from build123d import *

# Parameters (mm, degrees)
F1_DEPTH             = 20
F2_R                 = 5
F3_R                 = 1.99999
F6_D                 = 5
F6_DEPTH             = 10
F6_CSINK_D           = 10
F6_CSINK_ANGLE       = 90
F6_TIP               = 1.5021515476
F6_ON_F5_D           = 5
F6_ON_F5_DEPTH       = 10
F6_ON_F5_CSINK_D     = 10
F6_ON_F5_CSINK_ANGLE = 90
F6_ON_F5_TIP         = 1.5021515476
F7_D                 = 10
F7_DEPTH             = 49.0010001
F7_ON_F5_D           = 10
F7_ON_F5_DEPTH       = 49.0010001


# Not quite as in the source:
# - a fillet or chamfer is up to 0.001 mm smaller than in the source, because OpenCascade refuses the exact size


with BuildPart() as f1:
    # F0 (on Front) → F1 (new body, symmetric)
    with BuildSketch(Plane.XZ):
        with BuildLine():
            Line((44.5, 0), (-44, 0))
            Line((-44, 0), (-44, -9.25))
            Line((-44, -9.25), (0, -58.25))
            Line((0, -58.25), (46.5, -58.25))
            ThreePointArc((46.5, -58.25), (48.267766953, -57.517766953), (49, -55.75))
            ThreePointArc((49, -55.75), (48.267766953, -53.982233047), (46.5, -53.25))
            Line((46.5, -53.25), (5, -53.25))
            Line((5, -53.25), (5, -9.25))
            Line((5, -9.25), (44.5, -9.25))
            ThreePointArc((44.5, -9.25), (47.6819805153, -7.9319805153), (49, -4.75))
            Line((49, -4.75), (49, -4.5))
            ThreePointArc((49, -4.5), (47.6819805153, -1.3180194847), (44.5, 0))
        make_face()
        with BuildLine():
            Line((0, -52.2630996996), (-38.6240078935, -9.25))
            Line((-38.6240078935, -9.25), (-6, -9.25))
            ThreePointArc((-6, -9.25), (-1.7573593129, -11.0073593129), (0, -15.25))
            Line((0, -15.25), (0, -52.2630996996))
        make_face(mode=Mode.SUBTRACT)
    extrude(amount=F1_DEPTH, both=True)

    # F2
    f2_edges = [f1.edges().sort_by_distance(p)[0] for p in [
        (-44, 0, 0),
        (-44, 0, -9.25),
        (-38.624008, 0, -9.25),
        (0, 0, -52.2631),
        (0, 0, -58.25),
    ]]
    fillet(f2_edges, radius=F2_R)

    # F3 (radius 2 in the source; OpenCascade refuses exactly that, so slightly less here)
    f3_edges = [f1.edges().sort_by_distance(p)[0] for p in [
        (24.75, -20, -9.25),
        (25.75, -20, -53.25),
        (24.75, 20, -9.25),
        (-16.707111, -20, -9.25),
        (5, -20, -31.25),
        (5, 20, -31.25),
        (-16.707111, 20, -9.25),
    ]]
    fillet(f3_edges, radius=F3_R)

    # F6
    with Locations(Plane(origin=(0, 0, -9.25), x_dir=(1, 0, 0), z_dir=(0, 0, -1))):
        with Locations((24.75, 0)):
            CounterSinkHole(F6_D / 2, F6_CSINK_D / 2, depth=F6_DEPTH, counter_sink_angle=F6_CSINK_ANGLE)
            with Locations((0, 0, -(F6_DEPTH + F6_TIP / 2))):  # 118° drill point
                Cone(0, F6_D / 2, F6_TIP, mode=Mode.SUBTRACT)

    # F6 on F5
    with Locations(Plane(origin=(0, 0, -9.25), x_dir=(1, 0, 0), z_dir=(0, 0, -1))):
        with Locations((-16.7071109211, 0)):
            CounterSinkHole(F6_ON_F5_D / 2, F6_ON_F5_CSINK_D / 2, depth=F6_ON_F5_DEPTH, counter_sink_angle=F6_ON_F5_CSINK_ANGLE)
            with Locations((0, 0, -(F6_ON_F5_DEPTH + F6_ON_F5_TIP / 2))):  # 118° drill point
                Cone(0, F6_ON_F5_D / 2, F6_ON_F5_TIP, mode=Mode.SUBTRACT)

    # F7 (through all, one way)
    with BuildSketch(Plane.XY.offset(-9.25)):
        with Locations((24.75, 0)):
            Circle(F7_D / 2)
    extrude(amount=-F7_DEPTH, mode=Mode.SUBTRACT)

    # F7 on F5 (through all, one way)
    with BuildSketch(Plane.XY.offset(-9.25)):
        with Locations((-16.7071109211, 0)):
            Circle(F7_ON_F5_D / 2)
    extrude(amount=-F7_ON_F5_DEPTH, mode=Mode.SUBTRACT)


solid = f1.part
Input: part model. Units: mm. Frame: model coordinates. A direction names the side the tool comes from. Round coordinates to 2 decimals unless told otherwise and drop trailing zeros. Loops run counter-clockwise (first coordinate to the right, second up) from the corner with the lowest first, then second, coordinate; pieces in that order, holes last. Notation, with made-up numbers: (39.25, 79.5) -> (44.25, 79.5) arc R20 ccw to (44.25, 115.5) -> close; hole circle Ø8 at (46, 83). An arc over 180 degrees is marked (long way). Answer as a JSON object with one key per item and string values. Group by question number.
1) Section query D-D on y = 0. State how many separate pieces and enclosed holes the cut face has, plus the area to 3 significant figures.
2) Section query C-C on x = 42.5. Output: boundary loops of the cut face in (y, z).
3) Ray query, L1, parallel to Z at x = 25.5, y = -6.5; L2, parallel to Y at x = 24, z = -57. Return the intervals inside material, ascending.
4) Draft query along Z for faces 1 (the cylindrical face through (-15.3, -4.8, -36.5)), 2 (the flat face through (-22.261, -0.252, -27.473)), 3 (the cylindrical face through (47.717, -0.252, -1.353)), 4 (the flat face through (0, 0, -27)). Return one class per face: +Z half, -Z half, draft (parallel to the pull), parting line (faces both ways), or undercut.
5) Section query B-B on y = -15. Output: boundary loops of the cut face in (x, z), plus the area to 3 significant figures.
6) Reachability of faces 5 (the flat face through (5, 0, -32)), 6 (the cylindrical face through (-16.56, -19.43, -8.65)), 7 (the cylindrical face through (0.6, 19.43, -27.4)), 8 (the cylindrical face through (-1.804, -0.252, -10.961)), 9 (the cylindrical face through (24.04, 19.43, -8.65)) from +Z, -Z, +X, -X, +Y, -Y: full face, straight path, thin tool, end or side. Return the list, or none.
7) Section query A-A on x = 24.75. Output: boundary loops of the cut face in (y, z).
8) Pin query (flat end, axial travel): pin 1 (6 mm diameter, centred on y = -1.5, z = -28.5, fed in from -X); pin 2 (6 mm diameter, centred on y = -1.5, z = -47, fed in from -X); pin 3 (12 mm diameter, centred on y = 0.5, z = -30, fed in from -X); pin 4 (4 mm diameter, centred on x = -16.71, y = 0, fed in from +Z). Return the tip coordinate at first contact, or that it passes through.
Reply:
{
 "1": {"separate pieces": "4", "enclosed holes": "0", "area": "1,410 mm2"},
 "2": {"outline": "(-20, -56.25) arc R2 ccw to (-18, -58.25) -> (18, -58.25) arc R2 ccw to (20, -56.25) -> (20, -55.25) arc R2 ccw to (18, -53.25) -> (-18, -53.25) arc R2 ccw to (-20, -55.25) -> close; (-20, -7.25) arc R2 ccw to (-18, -9.25) -> (18, -9.25) arc R2 ccw to (20, -7.25) -> (20, -2) arc R2 ccw to (18, 0) -> (-18, 0) arc R2 ccw to (-20, -2) -> close"},
 "3": {"L1": "z = -58.25 to -53.25, -9.25 to 0", "L2": "y = -19.85 to -4.94, 4.94 to 19.85"},
 "4": {"face 1": "draft", "face 2": "undercut", "face 3": "+Z half", "face 4": "undercut"},
 "5": {"outline": "(-44, -7.33) arc R5 ccw to (-42.72, -10.68) -> (-1.49, -56.59) arc R5 ccw to (2.23, -58.25) -> (46.5, -58.25) arc R2.5 ccw to (46.5, -53.25) -> (5, -53.25) -> (5, -9.25) -> (44.5, -9.25) arc R4.5 ccw to (49, -4.75) -> (49, -4.5) arc R4.5 ccw to (44.5, 0) -> (-39, 0) arc R5 ccw to (-44, -5) -> close; hole (-31.13, -17.59) -> (-8.72, -42.55) arc R5 ccw to (0, -39.21) -> (0, -15.25) arc R6 ccw to (-6, -9.25) -> (-27.41, -9.25) arc R5 ccw to start", "area": "1,620 mm2"},
 "6": {"face 5": "+X, +Y, -Y", "face 6": "-Y", "face 7": "+Y", "face 8": "+Y, -Y", "face 9": "+X, +Y"},
 "7": {"outline": "(-20, -56.25) arc R2 ccw to (-18, -58.25) -> (-5, -58.25) -> (-5, -53.25) -> (-18, -53.25) arc R2 ccw to (-20, -55.25) -> close; (-20, -7.25) arc R2 ccw to (-18, -9.25) -> (-5, -9.25) -> (-2.5, -6.75) -> (-2.5, 0) -> (-18, 0) arc R2 ccw to (-20, -2) -> close; (2.5, -6.75) -> (5, -9.25) -> (18, -9.25) arc R2 ccw to (20, -7.25) -> (20, -2) arc R2 ccw to (18, 0) -> (2.5, 0) -> close; (5, -58.25) -> (18, -58.25) arc R2 ccw to (20, -56.25) -> (20, -55.25) arc R2 ccw to (18, -53.25) -> (5, -53.25) -> close"},
 "8": {"pin 1": "stops at x = -29.41", "pin 2": "stops at x = -12.54", "pin 3": "stops at x = -30.76", "pin 4": "passes through"}
}
